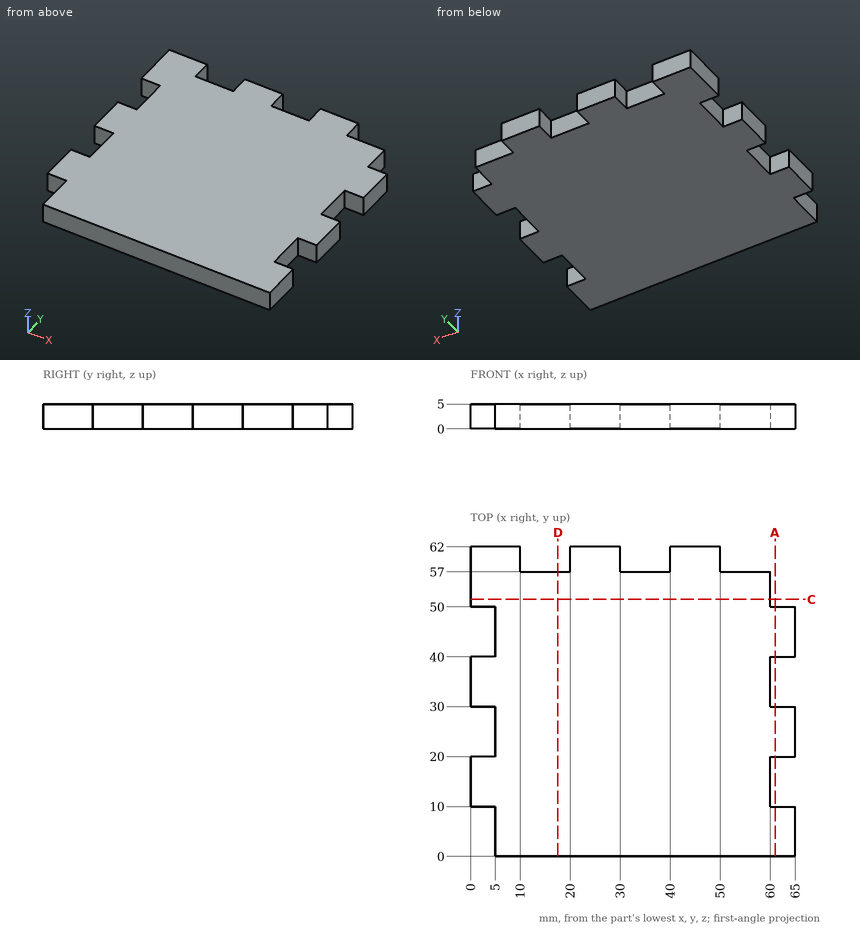
Design review of the part shown in the three views and the two pictorial views. Dimensions are in mm from the part's minimum x, y and z. Give positions to 0.01 mm unless a question says otherwise; leave off trailing zeros. Write each loop counter-clockwise with the first axis right and the second up, starting at its lowest first coordinate (ties: lowest second). Pieces come first, ordered by that corner, then holes. Notation, with made-up numbers: M -0.75,-38 L 21.25,-38 A19 ccw 21.25,-30 Z; hole C 51,12 d9. An arc over 180 degrees is marked long. One line per question, with ' | ' between items. Start each with the question number.
Item 1: We need section C-C on y = 51.5. Write out the cut boundary in (x, z), plus the area to 3 significant figures.
Item 2: Wall thickness on line 1 (X direction, y = 58.5, z = 4.05); line 2 (X direction, y = 37, z = 3.95); line 3 (Y direction, x = 59, z = 4.5): over which ranges is each line inside the solid? List them lowest first. Write a range as from..to.
Item 3: We need section A-A on x = 61. Write out the cut boundary in (y, z).
Item 4: We need section D-D on x = 17.5. Write out the cut boundary in (y, z), plus the area to 3 significant figures.
Item 5: For pin 1 (1.5 mm diameter, centred on y = 55, z = 2.5, fed in from +X); pin 2 (2.5 mm diameter, centred on x = 33, z = 1.5, fed in from +Y); pin 3 (2.5 mm diameter, centred on y = 27, z = 3.5, fed in from -X), all flat-tipped, find the tip position at first contact; note any pin that passes through.
Results found:
1) outline: M 0,0 L 60,0 L 60,5 L 0,5 Z | area: 300 mm2
2) line 1: x = 0..10, 20..30, 40..50 | line 2: x = 0..60 | line 3: y = 0..57
3) outline: M 0,0 L 10,0 L 10,5 L 0,5 Z; M 20,0 L 30,0 L 30,5 L 20,5 Z; M 40,0 L 50,0 L 50,5 L 40,5 Z
4) outline: M 0,0 L 57,0 L 57,5 L 0,5 Z | area: 285 mm2
5) pin 1: stops at x = 60 | pin 2: stops at y = 57 | pin 3: stops at x = 5
